```python
from build123d import *

# Parameters (mm, degrees)
SKETCH_W             = 1219.2
SKETCH_H             = 609.6
PAD_DEPTH            = 101.6
SKETCH001_W          = 1219.2
SKETCH001_H          = 558.8
PAD001_DEPTH         = 152.4
SKETCH002_W          = 508
SKETCH002_H          = 508
PAD002_DEPTH         = 127
BODY_PLACEMENT_ANGLE = 90


with BuildPart() as part:
    # Sketch → Pad (new body)
    with BuildSketch(Plane.XY):
        with Locations((609.6, 304.8)):
            Rectangle(SKETCH_W, SKETCH_H)
    extrude(amount=PAD_DEPTH)

    # Sketch001 (on Face6 of Pad) → Pad001 (join)
    with BuildSketch(Plane.XY.offset(101.6)):
        with Locations((609.6, 304.8)):
            Rectangle(SKETCH001_W, SKETCH001_H)
    extrude(amount=PAD001_DEPTH)

    # Sketch002 (on Face12 of Pad001) → Pad002 (join)
    with BuildSketch(Plane.XY.offset(254)):
        with Locations((609.6, 304.8)):
            Rectangle(SKETCH002_W, SKETCH002_H)
    extrude(amount=PAD002_DEPTH)


with BuildPart() as part_1:
    # Body placement: moved
    add(part.part.moved(Location((-307.6575, 1219.2, 2458.9105))).rotate(Axis((-307.6575, 1219.2, 2458.9105), (0, 0, 1)), BODY_PLACEMENT_ANGLE))


solid = part_1.part
```
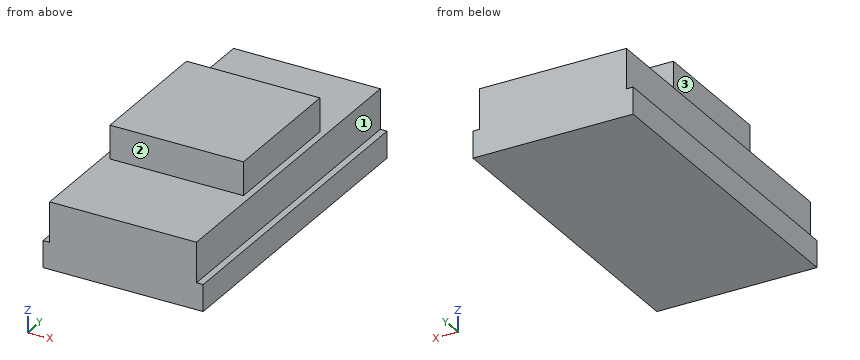
Input: part model. Units: mm. Frame: model coordinates. Face numbers are marked on the shaded views. A direction names the side the tool comes from. Give positions to 0.01 mm unless a question says otherwise; leave off trailing zeros. Order: outer loops, then holes, each group sorted by start corner. A loop starts at its lowest first (then second) coordinate and runs counter-clockwise, first axis right, second up. Notation, with made-up numbers: M 81.5,86.5 L 121.5,86.5 A26 ccw 121.5,109.5 Z; hole C 31,31.25 d2. An arc over 180 degrees is marked long. Return JSON: item names as keys, results as strings.
1) Section query A-A on x = -445. Output: boundary loops of the cut face in (y, z), and give its area (3 significant figures).
Taken from the geometry:
{"outline": "M 1219.2,2458.91 L 2438.4,2458.91 L 2438.4,2712.91 L 2082.8,2712.91 L 2082.8,2839.91 L 1574.8,2839.91 L 1574.8,2712.91 L 1219.2,2712.91 Z", "area": "374,000 mm2"}
2) Section query C-C on z = 2728. Output: boundary loops of the cut face in (x, y).
Taken from the geometry:
{"outline": "M -866.46,1574.8 L -358.46,1574.8 L -358.46,2082.8 L -866.46,2082.8 Z"}
3) Section query D-D on y = 2289.5. Output: boundary loops of the cut face in (x, z), and give its area (3 significant figures).
Taken from the geometry:
{"outline": "M -917.26,2458.91 L -307.66,2458.91 L -307.66,2560.51 L -333.06,2560.51 L -333.06,2712.91 L -891.86,2712.91 L -891.86,2560.51 L -917.26,2560.51 Z", "area": "147,000 mm2"}
4) Contact query for flat-ended pins moving along their axis: pin 1 (12 mm diameter, centred on y = 1969, z = 2783.5, fed in from +X); pin 2 (7.5 mm diameter, centred on x = -323.5, y = 1705.5, fed in from +Z); pin 3 (3 mm diameter, centred on y = 1650.5, z = 2711, fed in from +X). Output: stop coordinate, or through.
Taken from the geometry:
{"pin 1": "stops at x = -358.46", "pin 2": "stops at z = 2560.51", "pin 3": "stops at x = -333.06"}
5) Section query B-B on y = 1600. Output: boundary loops of the cut face in (x, z).
Taken from the geometry:
{"outline": "M -917.26,2458.91 L -307.66,2458.91 L -307.66,2560.51 L -333.06,2560.51 L -333.06,2712.91 L -358.46,2712.91 L -358.46,2839.91 L -866.46,2839.91 L -866.46,2712.91 L -891.86,2712.91 L -891.86,2560.51 L -917.26,2560.51 Z"}
6) Line query: L1, parallel to X at y = 1585.5, z = 2581; L2, parallel to Y at x = -508.5, z = 2737.5; L3, parallel to Z at x = -820, y = 2234. Output: solid intervals per line, ascending. Write a range as [from, to].
Taken from the geometry:
{"L1": "x = [-891.86, -333.06]", "L2": "y = [1574.8, 2082.8]", "L3": "z = [2458.91, 2712.91]"}
7) Access query for the marked faces 1, 2 and 3. Directions: +Z, -Z, +X, -X, +Y, -Y. A direction counts if a zero-diameter tool reaches every point of the face in a straight line with its end or side. Return the directions, or none.
Taken from the geometry:
{"face 1": "+Z, +X, +Y, -Y", "face 2": "+Z, +X, -X, -Y", "face 3": "+Z, -X, +Y, -Y"}
